from build123d import *

# Parameters (mm, degrees)
SKETCH_1_W      = 69
SKETCH_1_H      = 50
EXTRUDE_1_DEPTH = 4
SKETCH_2_R      = 1.6
EXTRUDE_2_DEPTH = 1.2
SKETCH_3_W      = 6.5
SKETCH_3_H      = 41
EXTRUDE_3_DEPTH = 20


with BuildPart() as part:
    # 草图1 → 凸台-拉伸1 (new body)
    with BuildSketch(Plane.XY):
        with Locations((34.5, 25)):
            Rectangle(SKETCH_1_W, SKETCH_1_H)
    extrude(amount=EXTRUDE_1_DEPTH)

    # 草图2 → 凸台-拉伸2 (add)
    with BuildSketch(Plane.XY.offset(4)):
        with BuildLine():
            Line((-5, 51), (74, 51))
            ThreePointArc((74, 51), (75.414213562, 50.414213562), (76, 49))
            Line((76, 49), (76, 1))
            ThreePointArc((76, 1), (75.414213562, -0.414213562), (74, -1))
            Line((74, -1), (-5, -1))
            ThreePointArc((-5, -1), (-6.414213562, -0.414213562), (-7, 1))
            Line((-7, 1), (-7, 49))
            ThreePointArc((-7, 49), (-6.414213562, 50.414213562), (-5, 51))
        make_face()
        with Locations((-4.3, 48.3)):
            Circle(SKETCH_2_R, mode=Mode.SUBTRACT)
        with Locations((73.3, 48.3)):
            Circle(SKETCH_2_R, mode=Mode.SUBTRACT)
        with Locations((-4.3, 1.7)):
            Circle(SKETCH_2_R, mode=Mode.SUBTRACT)
        with Locations((73.3, 1.7)):
            Circle(SKETCH_2_R, mode=Mode.SUBTRACT)
    extrude(amount=EXTRUDE_2_DEPTH)

    # 草图3 → 凸台-拉伸3 (add)
    with BuildSketch(Plane.XY.offset(5.2)):
        with Locations((-3.55, 25)):
            Rectangle(SKETCH_3_W, SKETCH_3_H)
    extrude(amount=EXTRUDE_3_DEPTH)


solid = part.part
Here's how the part is built. I have some questions about the finished solid (model axes, mm). A direction names the side the tool comes from. Coordinates: 2 decimals unless noted, no trailing zeros. Loops run counter-clockwise (first coordinate to the right, second up) from the corner with the lowest first, then second, coordinate; pieces in that order, holes last. Notation, with made-up numbers: (24, 84) -> (75, 84) arc R28 ccw to (75, 120) -> close; hole circle Ø4 at (-37.75, 25.25). An arc over 180 degrees is marked (long way). Use one line per item in the form item = value. Start each with the question number.
(1) If we section it at A-A (y = 24): Please give me the cut outline in (x, z), then the cut area to 3 significant figures.
(2) If we section it at C-C (z = 11.5): Please give me the cut outline in (x, y), then the cut area to 4 significant figures.
(3) Please list where these lines run through material, in increasing order: line 1 along Y through (x, z) = (-4.3, 4.8); line 2 along X through (y, z) = (48.5, 4.75); line 3 along Z through (x, y) = (42.5, 17.5).
(4) If we section it at B-B (x = 7.5): Please give me the cut outline in (y, z).
(5) On a 3-axis mill with a long thin cutter (end or side, diameter ignored), from which of +Z, -Z, +X, -X, +Y, -Y can I reach the whole of each face in a straight line? I mean faces 4 (the face through (69, 25, 2)), 5 (the face through (-4, 45.5, 15)), 6 (the face through (0, 25, 2)). Say none if no direction works.
(6) Will these pins go through, and if not, where does the flat tip stop? pin 1 (4 mm diameter, centred on x = -4.3, y = 48.3, fed in from +Z); pin 2 (3.5 mm diameter, centred on x = 73.3, y = 48.3, fed in from -Z); pin 3 (1.2 mm diameter, centred on x = 32, z = 2.5, fed in from +Y).
(7) We'd pull the mould along X, two halves only. Please class faces 1 (the face through (-0.3, 25, 15)), 2 (the face through (34.7, 50.2, 4)), 3 (the face through (74.78, 47.69, 4.59)): pulls with the +X half, pulls with the -X half, needs draft (parallel to the pull), parting line crosses it, or undercut.
Verdict:
q1.outline = (-7, 4) -> (0, 4) -> (0, 0) -> (69, 0) -> (69, 4) -> (76, 4) -> (76, 5.2) -> (-0.3, 5.2) -> (-0.3, 25.2) -> (-6.8, 25.2) -> (-6.8, 5.2) -> (-7, 5.2) -> close
q1.area = 506 mm²
q2.outline = (-6.8, 4.5) -> (-0.3, 4.5) -> (-0.3, 45.5) -> (-6.8, 45.5) -> close
q2.area = 266.5 mm²
q3.line_1 = -1 to 0.1, 3.3 to 46.7, 49.9 to 51
q3.line_2 = -7 to -5.89, -2.71 to 71.71, 74.89 to 76
q3.line_3 = 0 to 5.2
q4.outline = (-1, 4) -> (0, 4) -> (0, 0) -> (50, 0) -> (50, 4) -> (51, 4) -> (51, 5.2) -> (-1, 5.2) -> close
q5.face_4 = -Z, +X, +Y, -Y
q5.face_5 = +Z, +X, -X, +Y
q5.face_6 = -Z, -X, +Y, -Y
q6.pin_1 = 5.2
q6.pin_2 = 4
q6.pin_3 = 50
q7.face_1 = pulls with the +X half
q7.face_2 = needs draft
q7.face_3 = undercut
